Geometry: final body of the model. Coordinates: model frame, mm. Face numbers are marked on the shaded views. A direction names the side the tool comes from. Coordinates: 2 decimals unless noted, no trailing zeros. Order: outer loops, then holes, each group sorted by start corner. A loop starts at its lowest first (then second) coordinate and runs counter-clockwise, first axis right, second up. Notation, with made-up numbers: M -34,71.5 L 1,71.5 A31 cw 1,100.5 Z; hole C -17,42.25 d7. An arc over 180 degrees is marked long. Use CSV: the item, a comma, the result in double quotes. Start each with the question number.
1. Material intervals for line 1 (Z direction, x = 7, y = 7.3); line 2 (X direction, y = 7.55, z = 24); line 3 (X direction, y = 0.75, z = 47), sorted ascending.
2. Section query B-B on z = 3. Return the cut outline in (x, y), and give its area (3 significant figures).
3. Section query A-A on x = 0. Return the cut outline in (y, z).
4. First-contact query: P1, Ø6, axis at x = 5, z = 32.5, coming from the +Y side; P2, Ø1.5, axis at x = 2.5, z = 31, coming from the -Y side; P3, Ø2, axis at x = -2, y = 3, coming from the +Z side; P4, Ø8, axis at x = 7, z = 24, coming from the -Y side. Flat tips, straight axial feed; report the tip coordinate or a pass-through.
5. Section query C-C on y = 7.25. Return the cut outline in (x, z), and give its area (3 significant figures).
6. Set-up query: the marked faces 1 and 2. Return all of +Z, -Z, +X, -X, +Y, -Y with unobstructed straight access to the full face (end or side cutting, diameter ignored); none if empty.
7. Section query D-D on x = 7. Return the cut outline in (y, z).
8. Pull-direction query (Y, two-part tool) for the marked faces 3, 4 and 5; classes: pulls with the +Y half, pulls with the -Y half, needs draft (parallel to the pull), parting line crosses it, or undercut.
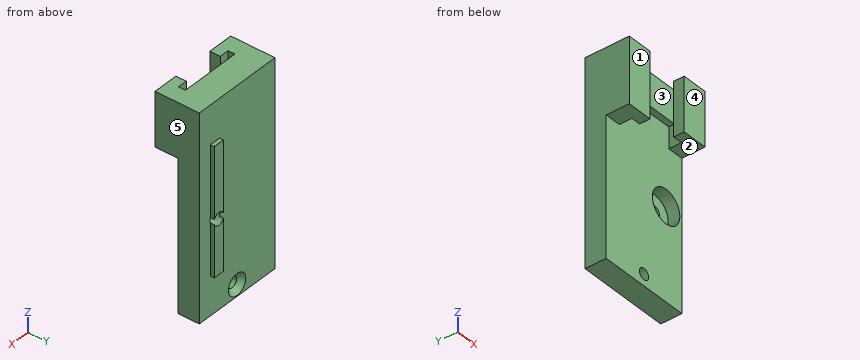
from build123d import *

# Parameters (mm, degrees)
MAIN_DEPTH                                        = 53
SKETCH2_W                                         = 24
SKETCH2_H                                         = 36
CUT_EXTRUDE1_DEPTH                                = 6
SKETCH3_W                                         = 2.9
SKETCH3_H                                         = 33
MAKERBEAMRAIL_DEPTH                               = 1
SKETCH4_R                                         = 1.6
MAKERBEAMHOLE_DEPTH                               = 13.5
SKETCH5_R                                         = 4.35
MAKERBEAMBIGHOLE_DEPTH                            = 3
SKETCH6_W                                         = 15.7
SKETCH6_H                                         = 8.5
PINHOLES_DEPTH                                    = 1.5
CSK_FOR_M2_5_FLAT_HEAD_MACHINE_SCREW1_D           = 2.9
CSK_FOR_M2_5_FLAT_HEAD_MACHINE_SCREW1_CSINK_D     = 5.5
CSK_FOR_M2_5_FLAT_HEAD_MACHINE_SCREW1_CSINK_ANGLE = 90
SKETCH9_W                                         = 6.6
SKETCH9_H                                         = 3
CUT_EXTRUDE5_DEPTH                                = 6


with BuildPart() as part:
    # Sketch1 → Main (new body)
    with BuildSketch(Plane.XY):
        Polygon((12, 0), (5.4, 0), (5.4, 2.7), (7.85, 2.7), (7.85, 4.5), (-7.85, 4.5), (-7.85, 2.7), (-5.4, 2.7), (-5.4, 0), (-12, 0), (-12, 11.5), (12, 11.5), align=None)
    extrude(amount=MAIN_DEPTH)

    # Sketch2 → Cut-Extrude1 (cut)
    with BuildSketch(Plane(origin=(0, 0, 0), x_dir=(1, 0, 0), z_dir=(0, 1, 0))):
        with Locations((0, -18)):
            Rectangle(SKETCH2_W, SKETCH2_H)
    extrude(amount=CUT_EXTRUDE1_DEPTH, mode=Mode.SUBTRACT)

    # Sketch3 → MakerBeamRail (add)
    with BuildSketch(Plane(origin=(0, 11.5, 0), x_dir=(1, 0, 0), z_dir=(0, 1, 0))):
        with Locations((7, -26.5)):
            Rectangle(SKETCH3_W, SKETCH3_H)
    extrude(amount=MAKERBEAMRAIL_DEPTH)

    # Sketch4 → MakerBeamHole (cut, through all)
    with BuildSketch(Plane(origin=(0, 12.5, 0), x_dir=(1, 0, 0), z_dir=(0, 1, 0))):
        with Locations((7, -24)):
            Circle(SKETCH4_R)
    extrude(amount=-MAKERBEAMHOLE_DEPTH, mode=Mode.SUBTRACT)

    # Sketch5 → MakerBeamBigHole (cut)
    with BuildSketch(Plane(origin=(0, 6, 0), x_dir=(-1, 0, 0), z_dir=(0, -1, 0))):
        with Locations((-7, -24)):
            Circle(SKETCH5_R)
    extrude(amount=-MAKERBEAMBIGHOLE_DEPTH, mode=Mode.SUBTRACT)

    # Sketch6 → PinHoles (cut)
    with BuildSketch(Plane.XZ.offset(-4.5)):
        with Locations((0, 40.25)):
            Rectangle(SKETCH6_W, SKETCH6_H)
    extrude(amount=-PINHOLES_DEPTH, mode=Mode.SUBTRACT)

    # CSK for M2.5 Flat Head Machine Screw1 (through all)
    with Locations(Plane(origin=(0, 11.5, 0), x_dir=(1, 0, 0), z_dir=(0, 1, 0))):
        with Locations((0, -3)):
            CounterSinkHole(CSK_FOR_M2_5_FLAT_HEAD_MACHINE_SCREW1_D / 2, CSK_FOR_M2_5_FLAT_HEAD_MACHINE_SCREW1_CSINK_D / 2, counter_sink_angle=CSK_FOR_M2_5_FLAT_HEAD_MACHINE_SCREW1_CSINK_ANGLE)

    # Sketch9 → Cut-Extrude5 (cut)
    with BuildSketch(Plane(origin=(0, 0, 0), x_dir=(-1, 0, 0), z_dir=(0, -1, 0))):
        with Locations((-8.7, -37.5)):
            Rectangle(SKETCH9_W, SKETCH9_H)
    extrude(amount=-CUT_EXTRUDE5_DEPTH, mode=Mode.SUBTRACT)


solid = part.part
Results list:
1,line 1,"z = 0 to 19.65, 28.35 to 53"
1,line 2,"x = -12 to 2.65, 11.35 to 12"
1,line 3,"x = -12 to -5.4, 5.4 to 12"
2,outline,"M -12,6 L -1.45,6 L -1.45,10.2 L -2.75,11.5 L -12,11.5 Z; M 1.45,6 L 12,6 L 12,11.5 L 2.75,11.5 L 1.45,10.2 Z"
2,area,"114 mm²"
3,outline,"M 4.5,44.5 L 6,44.5 L 6,4.45 L 10.2,4.45 L 11.5,5.75 L 11.5,53 L 4.5,53 Z; M 6,0 L 11.5,0 L 11.5,0.25 L 10.2,1.55 L 6,1.55 Z"
4,P1,"stops at y = 12.5"
4,P2,"stops at y = 6"
4,P3,"passes through"
4,P4,"stops at y = 9"
5,outline,"M -12,0 L 12,0 L 12,53 L -12,53 Z; hole C 0,3 d2.9; hole C 7,24 d8.7"
5,area,"1,210 mm²"
6,face 1,"+Z, -Z, +X, -X, -Y"
6,face 2,"-Z, +X, -Y"
7,outline,"M 0,39 L 2.7,39 L 2.7,53 L 0,53 Z; M 4.5,44.5 L 6,44.5 L 6,28.35 L 9,28.35 L 9,25.6 L 12.5,25.6 L 12.5,43 L 11.5,43 L 11.5,53 L 4.5,53 Z; M 6,0 L 11.5,0 L 11.5,10 L 12.5,10 L 12.5,22.4 L 9,22.4 L 9,19.65 L 6,19.65 Z"
8,face 3,"undercut"
8,face 4,"pulls with the -Y half"
8,face 5,"needs draft"
